from build123d import *

# Parameters (mm, degrees)
SKETCH2_W          = 0.5
SKETCH2_H          = 5
CUT_EXTRUDE1_DEPTH = 14.630480549
CIRPATTERN1_COUNT  = 2
CIRPATTERN1_ANGLE  = 90
CHAMFER1_SIZE2     = 1.5
CHAMFER1_SIZE      = 1.990567232
CHAMFER2_SIZE      = 1
CHAMFER2_SIZE2     = 1.37638192
CHAMFER3_SIZE      = 0.5


with BuildPart() as part:
    # Sketch1 → Revolve1 (revolve)
    with BuildSketch(Plane.XY, mode=Mode.PRIVATE) as revolve1_sk:
        Polygon((0, -8), (2, -8), (2, 0), (3.5, 0), (3.5, 9), (2, 9), (2, 12.7), (0, 12.7), align=None)
    revolve(revolve1_sk.sketch.rotate(Axis((0, -11.082621068, 0), (0, 1, 0)), 90), axis=Axis((0, -11.082621068, 0), (0, 1, 0)))

    # Sketch2 → Cut-Extrude1 (cut, symmetric)
    with BuildSketch(Plane.XY):
        with Locations((-3.25, 3.5)):
            Rectangle(SKETCH2_W, SKETCH2_H)
        with Locations((3.25, 3.5)):
            Rectangle(SKETCH2_W, SKETCH2_H)
    cut_extrude1 = extrude(amount=CUT_EXTRUDE1_DEPTH, both=True, mode=Mode.SUBTRACT)

    # CirPattern1: Cut-Extrude1 ×2 about axis
    cirpattern1_axis = Axis((0, -11.082621068, 0), (0, -1, 0))
    for i in range(1, CIRPATTERN1_COUNT):
        add(cut_extrude1.rotate(cirpattern1_axis, i * CIRPATTERN1_ANGLE / (CIRPATTERN1_COUNT - 1)), mode=Mode.SUBTRACT)

    # Chamfer1
    chamfer1_edges = [part.edges().sort_by_distance(p)[0] for p in [
        (0, 9, 3.5),
    ]]
    chamfer1_side = [part.faces().sort_by_distance(p)[0] for p in [
        (0, 8.97, 3.5),
    ]]
    chamfer(chamfer1_edges, length=CHAMFER1_SIZE - 0.0001, length2=CHAMFER1_SIZE2 - 0.0001, reference=chamfer1_side[0])  # a hair under: the kernel refuses the full size

    # Chamfer2
    chamfer2_edges = [part.edges().sort_by_distance(p)[0] for p in [
        (0, 12.7, 2),
    ]]
    chamfer2_side = [part.faces().sort_by_distance(p)[0] for p in [
        (0, 12.7, 0),
    ]]
    chamfer(chamfer2_edges, length=CHAMFER2_SIZE, length2=CHAMFER2_SIZE2, reference=chamfer2_side[0])

    # Chamfer3
    chamfer3_edges = [part.edges().sort_by_distance(p)[0] for p in [
        (0, -8, 2),
    ]]
    chamfer(chamfer3_edges, length=CHAMFER3_SIZE)


solid = part.part
Verification items for the finished model (mm, model axes). A direction names the side the tool comes from. Give positions to 0.01 mm unless a question says otherwise; leave off trailing zeros. Loops run counter-clockwise (first coordinate to the right, second up) from the corner with the lowest first, then second, coordinate; pieces in that order, holes last.
1) Depth check by flat-ended pin: pin 1 Ø4 at (x, y) = (1.5, 7) entering from -Z; pin 2 Ø1.8 at (x, y) = (0, 4.5) entering from +Z; pin 3 Ø1.8 at (y, z) = (2.5, 0.5) entering from +X; pin 4 Ø1.8 at (x, y) = (-0.5, 2.5) entering from -Z. Enter the tip coordinate at first touch or a pass-through.
2) Sectioned sample at D-D, the plane y = -4.5. Enter the section's corners in (x, z).
3) Set-up check for faces 5 (the flat face through (-3, 3, 0)), 6 (the flat face through (0, 3, 3)), 7 (the cylindrical face through (2, -4, 0)): record each of +Z, -Z, +X, -X, +Y, -Y from which the full face is reachable in a straight line by a thin tool's end or side.
4) Draft check along Y on faces 1 (the cylindrical face through (2, 10, 0)), 2 (the flat face through (2, 0, 2)), 3 (the flat face through (3, 3, 0)), 4 (the flat face through (0, 3, -3)). Enter one of: pulls with the +Y half, pulls with the -Y half, needs draft (parallel to the pull), parting line crosses it, or undercut.
5) Sectioned sample at A-A, the plane y = 2.25. Enter the section's corners in (x, z), then the cut area to 3 significant figures.
6) Thickness scan on line 1 along Z through (x, y) = (-1.5, 4); line 2 along X through (y, z) = (-4.75, 0). Record the ranges inside material, lowest first.
Answers:
1. pin 1: stops at z = -3.5
1. pin 2: stops at z = 3
1. pin 3: stops at x = 3
1. pin 4: stops at z = -3
2. outline: circle Ø4 at (0, 0)
3. face 5: +Z, -Z, -X
3. face 6: +Z, +X, -X
3. face 7: -Y
4. face 1: needs draft
4. face 2: pulls with the -Y half
4. face 3: undercut
4. face 4: undercut
5. outline: (-3, -1.8) arc R3.5 ccw to (-1.8, -3) - (1.8, -3) arc R3.5 ccw to (3, -1.8) - (3, 1.8) arc R3.5 ccw to (1.8, 3) - (-1.8, 3) arc R3.5 ccw to (-3, 1.8) - close
5. area: 33.6 mm2
6. line 1: z = -3 to 3
6. line 2: x = -2 to 2
